The listing builds one solid part. Answer for the finished solid, in the listing's coordinates (mm). Round coordinates to 2 decimals unless told otherwise and drop trailing zeros. Loops run counter-clockwise (first coordinate to the right, second up) from the corner with the lowest first, then second, coordinate; pieces in that order, holes last. Notation, with made-up numbers: (-21, 82.25) -> (28, 82.25) arc R25 ccw to (28, 107.25) -> close; hole circle Ø10 at (33, -19.5). An arc over 180 degrees is marked (long way). One line per question, with ' | ' between items.
Autodesk Inventor part; units mm, degrees
ref_plane "YZ Plane" through (0, 0, 0) normal (1, 0, 0) x (0, 1, 0)
ref_plane "XZ Plane" through (0, 0, 0) normal (0, 1, 0) x (-1, 0, 0)
ref_plane "XY Plane" through (0, 0, 0) normal (0, 0, 1) x (1, 0, 0)
sketch "Szkic1" plane through (0, 0, 0) normal (0, 0, 1) x (1, 0, 0)
  circle A0 centre (0, 0) radius 12.5
  line L0 (-35, 29) -> (35, 29)
  line L1 (35, -29) -> (-35, -29)
  line L2 (-35, 29) -> (-35, -29)
  line L3 (35, 29) -> (35, -29)
  dimension "d0" = 25
extrude "Wyciągnięcie proste1" add sketch "Szkic1" along normal blind 10
properties part number "rama_1"
Q1. Find the intervals of material crossed by line 1 (Y direction, x = 0, z = 6.5); line 2 (X direction, y = 10.5, z = 7); line 3 (Y direction, x = 2.5, z = 4.25), in increasing order. Write a range as from..to.
Numbers:
line 1: -29..-12.5, 12.5..29 | line 2: -35..-6.78, 6.78..35 | line 3: -29..-12.25, 12.25..29
Q2. A cutting plane is placed at A-A on y = 0. Give the vertices of the cut face in (x, z), plus the area to 3 significant figures.
Numbers:
outline: (-35, 0) -> (-12.5, 0) -> (-12.5, 10) -> (-35, 10) -> close; (12.5, 0) -> (35, 0) -> (35, 10) -> (12.5, 10) -> close | area: 450 mm^2
Q3. A cutting plane is placed at B-B on z = 1.5. Give the vertices of the cut face in (x, y).
Numbers:
outline: (-35, -29) -> (35, -29) -> (35, 29) -> (-35, 29) -> close; hole circle Ø25 at (0, 0)
Q4. A cutting plane is placed at C-C on x = 0. Give the vertices of the cut face in (y, z), plus the area to 3 significant figures.
Numbers:
outline: (-29, 0) -> (-12.5, 0) -> (-12.5, 10) -> (-29, 10) -> close; (12.5, 0) -> (29, 0) -> (29, 10) -> (12.5, 10) -> close | area: 330 mm^2
Q5. For a pull along X with two mould halves and no side action, classify faces 1 (the face through (-35, 0, 5)), 2 (the face through (11.923, -3.755, 4.93)), 3 (the face through (0, 13, 10)), 4 (the face through (35, 0, 5)) as pulls with the +X half, pulls with the -X half, needs draft (parallel to the pull), parting line crosses it, or undercut.
Numbers:
face 1: pulls with the -X half | face 2: undercut | face 3: needs draft | face 4: pulls with the +X half
